Can you work these out from the model? Positions are in its coordinate system, mm. Face numbers are marked on the shaded views. A direction names the side the tool comes from. Give positions to 0.01 mm unless a question says otherwise; leave off trailing zeros. Loops run counter-clockwise (first coordinate to the right, second up) from the corner with the lowest first, then second, coordinate; pieces in that order, holes last. Notation, with made-up numbers: M 83,45.5 L 105,45.5 A28 ccw 105,65.5 Z; hole C 2.25,81 d8. An arc over 180 degrees is marked long. Answer as a JSON object with one key per item and string values.
```python
from build123d import *

# Parameters (mm, degrees)
ESQUISSE1_R             = 2.4
BOSS_EXTRU_1_DEPTH      = 3
BOSS_EXTRU_2_DEPTH      = 3
ESQUISSE3_W             = 12
ESQUISSE3_H             = 25
ESQUISSE3_R             = 1.75
BOSS_EXTRU_3_DEPTH      = 3
ENL_V_MAT_EXTRU_1_DEPTH = 1.5
CONG_1_R                = 10


with BuildPart() as part:
    # Esquisse1 → Boss.-Extru.1 (new body)
    with BuildSketch(Plane(origin=(0, 0, 0), x_dir=(0, 0, -1), z_dir=(1, 0, 0))):
        Circle(ESQUISSE1_R)
    extrude(amount=BOSS_EXTRU_1_DEPTH)

    # Esquisse2 → Boss.-Extru.2 (add)
    with BuildSketch(Plane(origin=(3, 0, 0), x_dir=(0, 0, -1), z_dir=(1, 0, 0))):
        with BuildLine():
            Line((-2.4, 0), (-2.4, -10))
            Line((-2.4, -10), (2.4, -10))
            Line((2.4, -10), (2.4, 0))
            ThreePointArc((2.4, 0), (0, 2.4), (-2.4, 0))
        make_face()
    extrude(amount=BOSS_EXTRU_2_DEPTH)

    # Esquisse3 → Boss.-Extru.3 (add)
    with BuildSketch(Plane.XZ.offset(10)):
        with Locations((0, -10.1)):
            Rectangle(ESQUISSE3_W, ESQUISSE3_H)
        with Locations(Location((-1.75, -9.6, 0), (0, 0, 270))):
            Circle(ESQUISSE3_R, mode=Mode.SUBTRACT)
        with Locations(Location((-1.75, -17.6, 0), (0, 0, 270))):
            Circle(ESQUISSE3_R, mode=Mode.SUBTRACT)
    extrude(amount=BOSS_EXTRU_3_DEPTH)

    # Esquisse4 → Enlèv. mat.-Extru.1 (cut)
    with BuildSketch(Plane(origin=(0, -10, 0), x_dir=(1, 0, 0), z_dir=(0, 1, 0))):
        Polygon((-4.6, 7.954551733), (-4.6, 11.245448267), (-1.75, 12.890896534), (1.1, 11.245448267), (1.1, 7.954551733), (-1.75, 6.309103466), align=None)
        Polygon((-4.6, 15.954551733), (-4.6, 19.245448267), (-1.75, 20.890896534), (1.1, 19.245448267), (1.1, 15.954551733), (-1.75, 14.309103466), align=None)
    extrude(amount=-ENL_V_MAT_EXTRU_1_DEPTH, mode=Mode.SUBTRACT)

    # Congé1
    cong_1_edges = [part.edges().sort_by_distance(p)[0] for p in [
        (4.5, -10, -2.4),
    ]]
    fillet(cong_1_edges, radius=CONG_1_R - 0.0001)  # a hair under: the kernel refuses the full size


solid = part.part
```
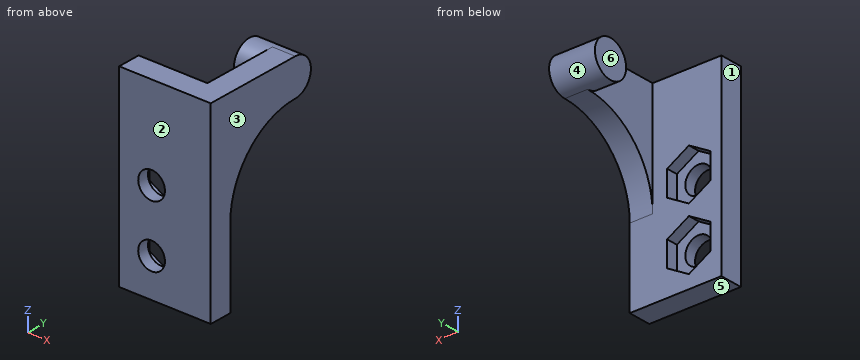
1) Will these pins go through, and if not, where does the flat tip stop? pin 1 Ø5 at (y, z) = (-6, -10) entering from +X; pin 2 Ø5 at (x, z) = (0, -17) entering from +Y; pin 3 Ø5.5 at (y, z) = (-1, -1) entering from -X; pin 4 Ø1.7 at (x, z) = (-1.5, -8.5) entering from +Y.
Answer list:
{"pin 1": "through", "pin 2": "y = -10", "pin 3": "x = 0", "pin 4": "y = -11.5"}
2) If we mould it in two halves opening along X, with no side actions, what happens to the marked faces 1, 2 and 3? For each: +X half, -X half, draft (parallel to the pull), parting line (faces both ways), or undercut.
Answer list:
{"face 1": "-X half", "face 2": "draft", "face 3": "+X half"}
3) Suppose I cut it at A-A, the plane z = -17.6. Write out the boundary of the cut face in (x, y).
Answer list:
{"outline": "M -6,-13 L -3.5,-13 L -3.5,-11.5 L -4.6,-11.5 L -4.6,-10 L -6,-10 Z; M 0,-13 L 6,-13 L 6,-10 L 1.1,-10 L 1.1,-11.5 L 0,-11.5 Z"}
4) Suppose I cut it at C-C, the plane x = -0.5. Write out the boundary of the cut face in (y, z), and give its area (3 significant figures).
Answer list:
{"outline": "M -13,-22.6 L -10,-22.6 L -10,-20.17 L -11.5,-20.17 L -11.5,-18.82 L -13,-18.82 Z; M -13,-16.38 L -11.5,-16.38 L -11.5,-15.03 L -10,-15.03 L -10,-12.17 L -11.5,-12.17 L -11.5,-10.82 L -13,-10.82 Z; M -13,-8.38 L -11.5,-8.38 L -11.5,-7.03 L -10,-7.03 L -10,2.4 L -13,2.4 Z", "area": "52.2 mm^2"}
5) Please list where these lines run through material, in increasing order: line 1 along Z through (x, y) = (-1.75, -12.1); line 2 along X through (y, z) = (-11.85, -17.6); line 3 along Y through (x, z) = (5, -18.25). Write a range as from..to.
Answer list:
{"line 1": "-22.6..-19.35, -15.85..-11.35, -7.85..2.4", "line 2": "-6..-3.5, 0..6", "line 3": "-13..-10"}
6) For the marked faces 4, 5 and 6, which set-ups out of +Z, -Z, +X, -X, +Y, -Y let a thin tool reach every point of the face, with its end or its side?
Answer list:
{"face 4": "-X", "face 5": "-Z, +X, -X, +Y, -Y", "face 6": "+Z, -Z, -X, +Y"}
7) Suppose I cut it at B-B, the plane z = 0. Write out the boundary of the cut face in (x, y), and give its area (3 significant figures).
Answer list:
{"outline": "M -6,-13 L 6,-13 L 6,2.4 L 0,2.4 L 0,-2.4 L 3,-2.4 L 3,-10 L -6,-10 Z", "area": "87.6 mm^2"}
